```python
from build123d import *

# Parameters (mm, degrees)
F0_W     = 254
F0_H     = 152.4
F1_DEPTH = 25.4
F2_R     = 22.688779
F3_W     = 228.6
F3_H     = 127
F4_DEPTH = 101.6


with BuildPart() as f1:
    # F0 (on Front) → F1 (new body)
    with BuildSketch(Plane.XZ):
        with Locations((-29.356187, 2.458728)):
            Rectangle(F0_W, F0_H)
    extrude(amount=F1_DEPTH)

    # F2
    f2_edges = [f1.edges().sort_by_distance(p)[0] for p in [
        (-29.356187, 0, 78.658728),
        (-156.356187, 0, 2.458728),
        (-29.356187, 0, -73.741272),
        (97.643813, 0, 2.458728),
    ]]
    fillet(f2_edges, radius=F2_R)

    # F3 (on face) → F4 (join)
    with BuildSketch(Plane.XZ.offset(25.4)):
        with Locations((-29.209957, 1.706252)):
            Rectangle(F3_W, F3_H)
    extrude(amount=F4_DEPTH)


solid = f1.part
```
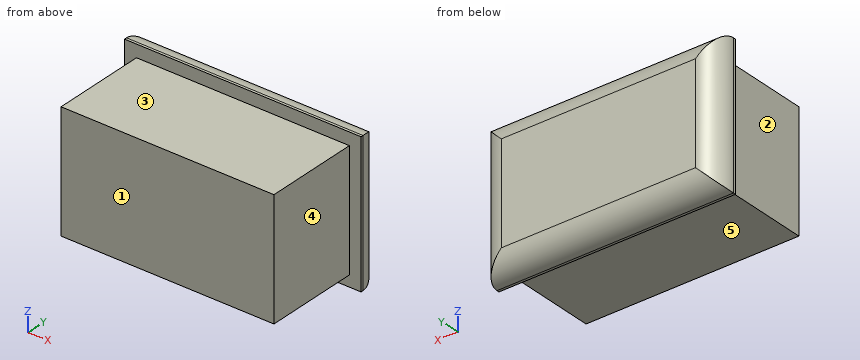
For this review, take the finished solid that the model builds, in its own axes (mm). Face numbers are marked on the shaded views. A direction names the side the tool comes from. Round coordinates to 2 decimals unless told otherwise and drop trailing zeros. Write each loop counter-clockwise with the first axis right and the second up, starting at its lowest first coordinate (ties: lowest second). Pieces come first, ordered by that corner, then holes. Notation, with made-up numbers: (45.5, 80.25) -> (89.5, 80.25) arc R18 cw to (89.5, 109.25) -> close; hole circle Ø6 at (46.25, 1.5). An arc over 180 degrees is marked (long way). Use one line per item in the form item = value.
Q1. Machinability: for the marked faces 1, 2, 3, 4 and 5, which of the approach directions +Z, -Z, +X, -X, +Y, -Y give a long, thin tool a straight path to every point of the face, cutting with its end or side? Answer none if there is none.
Resolved:
face_1 = +Z, -Z, +X, -X, -Y
face_2 = +Z, -Z, -X, -Y
face_3 = +Z, +X, -X, -Y
face_4 = +Z, -Z, +X, -Y
face_5 = -Z, +X, -X, -Y
Q2. Consider section C-C (y = -113). State the section outline as (x, z) points.
Resolved:
outline = (-143.51, -61.79) -> (85.09, -61.79) -> (85.09, 65.21) -> (-143.51, 65.21) -> close
Q3. Clearance check with flat-ended pins moving along their axes: pin 1 Ø1.5 at (y, z) = (-89.5, 52) entering from +X; pin 2 Ø12 at (x, y) = (63.5, -96.5) entering from +Z; pin 3 Ø3 at (x, y) = (-128.5, -19.5) entering from -Z. State where each tip first meets the part, or that it passes through.
Resolved:
pin_1 = 85.09
pin_2 = 65.21
pin_3 = -73.68
Q4. Consider section A-A (z = -44). State the section outline as (x, y) points, then the cut area to 3 significant figures.
Resolved:
outline = (-156.36, -25.4) -> (-143.51, -25.4) -> (-143.51, -127) -> (85.09, -127) -> (85.09, -25.4) -> (97.64, -25.4) -> (97.64, -22.69) arc R22.69 ccw to (74.96, 0) -> (-133.67, 0) arc R22.69 ccw to (-156.36, -22.69) -> close
area = 29,500 mm²
Q5. Consider section D-D (z = 68). State the section outline as (x, y) points.
Resolved:
outline = (-156.36, -25.4) -> (97.64, -25.4) -> (97.64, -22.69) arc R22.69 ccw to (86.99, -3.45) -> (-145.7, -3.45) arc R22.69 ccw to (-156.36, -22.69) -> close
Q6. Consider section B-B (x = -74.5). State the section outline as (y, z) points.
Resolved:
outline = (-127, -61.79) -> (-25.4, -61.79) -> (-25.4, -73.74) -> (-22.69, -73.74) arc R22.69 ccw to (0, -51.05) -> (0, 55.97) arc R22.69 ccw to (-22.69, 78.66) -> (-25.4, 78.66) -> (-25.4, 65.21) -> (-127, 65.21) -> close
Q7. To check wall thickness, follow probe 1 along X at (y, z) = (-69.5, -18.5); probe 2 along Z at (x, y) = (-94, -74.5); probe 3 along Z at (x, y) = (24.5, -18.5). State the ranges of each line that lie inside material, in increasing order. Write a range as from..to.
Resolved:
probe_1 = -143.51..85.09
probe_2 = -61.79..65.21
probe_3 = -73.35..78.27
